Here's how the part is built. I have some questions about the finished solid (model axes, mm). A direction names the side the tool comes from. Round coordinates to 2 decimals unless told otherwise and drop trailing zeros. Answer as a JSON object with one key per item and string values.
from build123d import *

# Parameters (mm, degrees)
F0_R     = 77.5
F0_R_2   = 62.5
F1_DEPTH = 9
F2_SIZE  = 5
F3_SIZE2 = 1.99999
F3_SIZE  = 8.99999
F4_R     = 5
F5_R     = 5
F6_DEPTH = 5
F7_R     = 2


# Not quite as in the source:
# - a fillet or chamfer is up to 0.001 mm smaller than in the source, because OpenCascade refuses the exact size


with BuildPart() as f1:
    # F0 (on Top) → F1 (new body)
    with BuildSketch(Plane.XY):
        Circle(F0_R)
        Circle(F0_R_2, mode=Mode.SUBTRACT)
    extrude(amount=F1_DEPTH)

    # F2
    f2_edges = [f1.edges().sort_by_distance(p)[0] for p in [
        (-77.5, 0, 9),
    ]]
    chamfer(f2_edges, length=F2_SIZE)

    # F3 (size 9 and 2 in the source; OpenCascade refuses exactly that, so slightly less here)
    f3_edges = [f1.edges().sort_by_distance(p)[0] for p in [
        (-62.5, 0, 9),
    ]]
    f3_side = f1.faces().sort_by_distance((-62.5, 0, 4.5))[0]
    chamfer(f3_edges, length=F3_SIZE, length2=F3_SIZE2, reference=f3_side)

    # F4
    f4_edges = [f1.edges().sort_by_distance(p)[0] for p in [
        (-64.49999, 0, 9),
    ]]
    fillet(f4_edges, radius=F4_R)

    # F5 (on face) → F6 (cut)
    with BuildSketch(Plane(origin=(0, 0, 0), x_dir=(1, 0, 0), z_dir=(0, 0, -1))):
        with Locations((0, 69)):
            Circle(F5_R)
        with Locations((-69, 0)):
            Circle(F5_R)
        with Locations((0, -69)):
            Circle(F5_R)
        with Locations((69, 0)):
            Circle(F5_R)
    extrude(amount=-F6_DEPTH, mode=Mode.SUBTRACT)

    # F7
    f7_edges = [f1.edges().sort_by_distance(p)[0] for p in [
        (-5, -69, 5),
        (-74, 0, 5),
        (64, 0, 5),
        (-5, 69, 5),
    ]]
    fillet(f7_edges, radius=F7_R)


solid = f1.part
Item 1: If we mould it in two halves opening along Y, with no side actions, what happens to faces 3 (the face through (69.38, 21.85, 8.76)), 4 (the face through (3, 65, 1)), 5 (the face through (0, -63, 0))? For each: pulls with the +Y half, pulls with the -Y half, needs draft (parallel to the pull), parting line crosses it, or undercut.
Resolved:
{"face 3": "parting line crosses it", "face 4": "undercut", "face 5": "needs draft"}
Item 2: Please list where these lines run through material, in increasing order: probe 1 along Y at (x, z) = (0, 2.4); probe 2 along Y at (x, z) = (0, 0.7); probe 3 along X at (y, z) = (12, 3.5). Write a range as from..to.
Resolved:
{"probe 1": "-77.5..-74, -64..-63.03, 63.03..64, 74..77.5", "probe 2": "-77.5..-74, -64..-62.66, 62.66..64, 74..77.5", "probe 3": "-76.57..-62.13, 62.13..76.57"}
Item 3: I'm going to push flat-ended pins straight in: pin 1 Ø4 at (y, z) = (13, 3.5) entering from -X; pin 2 Ø6.5 at (x, y) = (-69, 0) entering from -Z; pin 3 Ø1.5 at (x, z) = (1.5, 5.5) entering from +Y. Where does each tip first touch, or does it pass through?
Resolved:
{"pin 1": "x = -76.72", "pin 2": "z = 4.98", "pin 3": "y = 76.74"}
Item 4: On a 3-axis mill with a long thin cutter (end or side, diameter ignored), from which of +Z, -Z, +X, -X, +Y, -Y can I reach the whole of each face in a straight line? I mean faces 1 (the face through (-13.564, -61.083, 0.318)), 2 (the face through (73.619, 1.915, 1.479)). Say none if no direction works.
Resolved:
{"face 1": "+Z", "face 2": "-Z"}
